Build history of the part. All positions in model axes, mm. A direction names the side the tool comes from. Coordinates: 2 decimals unless noted, no trailing zeros. Order: outer loops, then holes, each group sorted by start corner. A loop starts at its lowest first (then second) coordinate and runs counter-clockwise, first axis right, second up. Notation, with made-up numbers: (-13.5, -34.5) - (21.5, -34.5) arc R21 cw to (21.5, -6.5) - close; hole circle Ø10 at (-36, -35.5). An arc over 180 degrees is marked (long way). Write each question's results on one line, items separated by ' | '. Start each with the question number.
from build123d import *

# Parameters (mm, degrees)
F1_DEPTH  = 80
F2_R      = 5
F3_DEPTH  = 25
F5_DEPTH  = 60
F6_R      = 35
F7_DEPTH  = 33.666907
F8_R      = 25
F9_DEPTH  = 52.6
F11_DEPTH = 25


with BuildPart() as f1:
    # F0 (on Front) → F1 (new body)
    with BuildSketch(Plane.XZ):
        Polygon((121, 0), (0, 0), (0, -15), (30, -15), (30, -10), (90, -10), (90, -15), (121, -15), align=None)
    extrude(amount=F1_DEPTH)

    # F2 (on face) → F3 (cut)
    with BuildSketch(Plane.XY):
        with Locations((15.5, -15)):
            Circle(F2_R)
        with Locations((15.5, -65)):
            Circle(F2_R)
        with Locations((105.5, -65)):
            Circle(F2_R)
        with Locations((105.5, -15)):
            Circle(F2_R)
    extrude(amount=-F3_DEPTH, mode=Mode.SUBTRACT)

    # F4 (on face) → F5 (join)
    with BuildSketch(Plane.XY):
        Polygon((34.5, -45), (81, -45), (81, -56.833453), (91, -56.833453), (91, -45), (91, -35), (91, -23.166547), (81, -23.166547), (81, -35), (34.5, -35), align=None)
    extrude(amount=F5_DEPTH)

    # F6 (on face) → F7 (join, through all)
    with BuildSketch(Plane.XZ.offset(56.833453)):
        with Locations((86, 60)):
            Circle(F6_R)
    extrude(amount=-F7_DEPTH)

    # F8 (on face) → F9 (cut)
    with BuildSketch(Plane.XZ.offset(56.833453)):
        with Locations((86, 60)):
            Circle(F8_R)
    extrude(amount=-F9_DEPTH, mode=Mode.SUBTRACT)

    # F10 (on face) → F11 (cut)
    with BuildSketch(Plane.XZ.offset(45)):
        Polygon((34.5, 60), (34.5, 0), (51, 60), align=None)
    extrude(amount=-F11_DEPTH, mode=Mode.SUBTRACT)


solid = f1.part
Item 1: Slice it at A-A (x = 15.5). Write the cut outline in (y, z).
Item 2: Slice it at D-D (z = 49.5). Write the cut outline in (x, y), then the cut area to 3 significant figures.
Item 3: Flat gauge pins, fed straight in: P1, Ø9.5, axis at y = -27.5, z = 17.5, coming from the -X side; P2, Ø14, axis at x = 62, z = 27, coming from the -Y side; P3, Ø8, axis at x = 73.5, y = -61.5, coming from the -Z side. Where does each tip first touch, or does it go through?
Item 4: Which spindle directions (+Z, -Z, +X, -X, +Y, -Y) get a long thin tool onto all of the face, cutting with end or side? Do faces 4 (the flat face through (81, -29, 13)), 5 (the flat face through (86, -56.833, 34)), 6 (the flat face through (86, -23.167, 13)), 7 (the flat face through (90, -39, -12)). Say none if no direction does.
Item 5: Probe probe 1 along X at (y, z) = (-14.5, -2.5); probe 2 along Y at (x, z) = (105.5, -10.5); probe 3 along Z at (x, y) = (86, -36). List the from-to ranges inside material, lowest first.
Item 6: Slice it at B-B (y = -15). Write the cut outline in (x, z), then the cut area to 4 significant figures.
Item 7: Pull direction X, two halves, no side cores. Call faces 1 (the cylindrical face through (110.119, -16.915, -7.395)), 2 (the flat face through (121, -39, -8)), 3 (the flat face through (15, -39, -15)): released by +X, released by -X, zero draft, split by the parting line, or undercut.
Resolved:
1) outline: (-80, -15) - (-70, -15) - (-70, 0) - (-80, 0) - close; (-60, -15) - (-20, -15) - (-20, 0) - (-60, 0) - close; (-10, -15) - (0, -15) - (0, 0) - (-10, 0) - close
2) outline: (48.11, -45) - (52.61, -45) - (52.61, -56.83) - (63.31, -56.83) - (63.31, -23.17) - (52.61, -23.17) - (52.61, -35) - (48.11, -35) - close; (108.69, -56.83) - (119.39, -56.83) - (119.39, -23.17) - (108.69, -23.17) - close | area: 765 mm^2
3) P1: x = 81 | P2: y = -56.83 | P3: z = -10
4) face 4: -X, +Y | face 5: +Z, +X, -X, -Y | face 6: +Z, +X, -X, +Y | face 7: -Z, +Y, -Y
5) probe 1: 0 to 10.53, 20.47 to 100.53, 110.47 to 121 | probe 2: -80 to -70, -60 to -20, -10 to 0 | probe 3: -10 to 35, 85 to 95
6) outline: (0, -15) - (10.5, -15) - (10.5, 0) - (0, 0) - close; (20.5, -15) - (30, -15) - (30, -10) - (90, -10) - (90, -15) - (100.5, -15) - (100.5, 0) - (20.5, 0) - close; (110.5, -15) - (121, -15) - (121, 0) - (110.5, 0) - close | area: 1,215 mm^2
7) face 1: undercut | face 2: released by +X | face 3: zero draft
